```python
from build123d import *

# Parameters (mm, degrees)
ESBO_O1_W                   = 131.4
ESBO_O1_H                   = 68.4
BASE_DEPTH                  = 1.2
FILETE1_R                   = 15
FILETE2_R                   = 15
FILETE3_R                   = 10
FILETE4_R                   = 10
PAREDES_START               = 15.5
PAREDES_DEPTH               = 15.5
ESBO_O6_R                   = 2.5
SUPORTE_DOS_PARAFUSOS_DEPTH = 15.5
ESBO_O7_R                   = 1.1
FURO_DOS_PARAFUSOS_DEPTH    = 6
FECHAMENTOS_REACH           = 77.928
ESBO_O14_W                  = 10
ESBO_O14_H                  = 4.5
CORTE_DO_USB_DEPTH          = 10
ESBO_O16_W                  = 15.2
ESBO_O16_H                  = 9.3
CORTE_DAS_CHAVES_DEPTH      = 10
ESBO_O17_W                  = 15
ESBO_O17_H                  = 6
CORTE_SD_DEPTH              = 10
CHANFRO_BASE_INTERIOR_SIZE  = 2
FILETE5_R                   = 2


with BuildPart() as part:
    # Esboço1 → Base (new body)
    with BuildSketch(Plane(origin=(0, 0, 0), x_dir=(1, 0, 0), z_dir=(0, 1, 0))):
        Rectangle(ESBO_O1_W, ESBO_O1_H)
    extrude(amount=BASE_DEPTH)

    # Filete1
    filete1_edges = [part.edges().sort_by_distance(p)[0] for p in [
        (65.7, 0.6, 34.2),
    ]]
    fillet(filete1_edges, radius=FILETE1_R)

    # Filete2
    filete2_edges = [part.edges().sort_by_distance(p)[0] for p in [
        (-65.7, 0.6, 34.2),
    ]]
    fillet(filete2_edges, radius=FILETE2_R)

    # Filete3
    filete3_edges = [part.edges().sort_by_distance(p)[0] for p in [
        (65.7, 0.6, -34.2),
    ]]
    fillet(filete3_edges, radius=FILETE3_R)

    # Filete4
    filete4_edges = [part.edges().sort_by_distance(p)[0] for p in [
        (-65.7, 0.6, -34.2),
    ]]
    fillet(filete4_edges, radius=FILETE4_R)

    # Esboço5 → Paredes (add)
    with BuildSketch(Plane(origin=(0, 1.2, 0), x_dir=(1, 0, 0), z_dir=(0, 1, 0)).offset(PAREDES_START)):
        with BuildLine():
            Line((55.7, 34.2), (-55.7, 34.2))
            ThreePointArc((-55.7, 34.2), (-62.771067812, 31.271067812), (-65.7, 24.2))
            Line((-65.7, 24.2), (-65.7, -19.2))
            ThreePointArc((-65.7, -19.2), (-61.306601718, -29.806601718), (-50.7, -34.2))
            Line((-50.7, -34.2), (50.7, -34.2))
            ThreePointArc((50.7, -34.2), (61.306601718, -29.806601718), (65.7, -19.2))
            Line((65.7, -19.2), (65.7, 24.2))
            ThreePointArc((65.7, 24.2), (62.771067812, 31.271067812), (55.7, 34.2))
        make_face()
        with BuildLine():
            Line((55.7, 33), (-55.7, 33))
            ThreePointArc((-55.7, 33), (-61.922539674, 30.422539674), (-64.5, 24.2))
            Line((-64.5, 24.2), (-64.5, -19.2))
            ThreePointArc((-64.5, -19.2), (-60.45807358, -28.95807358), (-50.7, -33))
            Line((-50.7, -33), (50.7, -33))
            ThreePointArc((50.7, -33), (60.45807358, -28.95807358), (64.5, -19.2))
            Line((64.5, -19.2), (64.5, 24.2))
            ThreePointArc((64.5, 24.2), (61.922539674, 30.422539674), (55.7, 33))
        make_face(mode=Mode.SUBTRACT)
    extrude(amount=-PAREDES_DEPTH)

    # Esboço6 → Suporte dos parafusos (add)
    with BuildSketch(Plane(origin=(0, 1.2, 0), x_dir=(1, 0, 0), z_dir=(0, 1, 0))):
        with Locations(Location((-59.7, 28.2, 0), (0, 0, 90))):
            Circle(ESBO_O6_R)
        with Locations(Location((-57.7, -26.2, 0), (0, 0, 90))):
            Circle(ESBO_O6_R)
        with Locations(Location((59.7, 28.2, 0), (0, 0, 90))):
            Circle(ESBO_O6_R)
        with Locations(Location((57.7, -26.2, 0), (0, 0, 90))):
            Circle(ESBO_O6_R)
    extrude(amount=SUPORTE_DOS_PARAFUSOS_DEPTH)

    # Esboço7 → Furo dos parafusos (cut)
    with BuildSketch(Plane(origin=(0, 16.7, 0), x_dir=(1, 0, 0), z_dir=(0, 1, 0))):
        with Locations(Location((-59.7, 28.2, 0), (0, 0, 270))):
            Circle(ESBO_O7_R)
        with Locations(Location((59.7, 28.2, 0), (0, 0, 270))):
            Circle(ESBO_O7_R)
        with Locations(Location((57.7, -26.2, 0), (0, 0, 270))):
            Circle(ESBO_O7_R)
        with Locations(Location((-57.7, -26.2, 0), (0, 0, 270))):
            Circle(ESBO_O7_R)
    extrude(amount=-FURO_DOS_PARAFUSOS_DEPTH, mode=Mode.SUBTRACT)

    # Esboço23 → Fechamentos (add, up to next)
    with BuildSketch(Plane(origin=(0, 16.7, 0), x_dir=(1, 0, 0), z_dir=(0, 1, 0)), mode=Mode.PRIVATE) as fechamentos_sk1:
        with BuildLine():
            Line((57.2, 28.2), (57.2, 32.871216754))
            ThreePointArc((57.2, 32.871216754), (61.922539674, 30.422539674), (64.371216754, 25.7))
            Line((64.371216754, 25.7), (59.7, 25.7))
            Line((59.7, 25.7), (62.2, 28.2))
            Line((62.2, 28.2), (59.7, 30.7))
            Line((59.7, 30.7), (57.2, 28.2))
        make_face()
    fechamentos_tool1 = extrude(fechamentos_sk1.sketch, amount=-FECHAMENTOS_REACH, mode=Mode.PRIVATE) - part.part
    # Esboço23 → Fechamentos (add, up to next)
    with BuildSketch(Plane(origin=(0, 16.7, 0), x_dir=(1, 0, 0), z_dir=(0, 1, 0)), mode=Mode.PRIVATE) as fechamentos_sk2:
        with BuildLine():
            Line((-59.7, 25.7), (-64.371216754, 25.7))
            ThreePointArc((-64.371216754, 25.7), (-61.922539674, 30.422539674), (-57.2, 32.871216754))
            Line((-57.2, 32.871216754), (-57.2, 28.2))
            Line((-57.2, 28.2), (-59.7, 30.7))
            Line((-59.7, 30.7), (-62.2, 28.2))
            Line((-62.2, 28.2), (-59.7, 25.7))
        make_face()
    fechamentos_tool2 = extrude(fechamentos_sk2.sketch, amount=-FECHAMENTOS_REACH, mode=Mode.PRIVATE) - part.part
    # Esboço23 → Fechamentos (add, up to next)
    with BuildSketch(Plane(origin=(0, 16.7, 0), x_dir=(1, 0, 0), z_dir=(0, 1, 0)), mode=Mode.PRIVATE) as fechamentos_sk3:
        with BuildLine():
            Line((57.7, -23.7), (63.745688943, -23.7))
            ThreePointArc((63.745688943, -23.7), (60.45807358, -28.95807358), (55.2, -32.245688943))
            Line((55.2, -32.245688943), (55.2, -26.2))
            Line((55.2, -26.2), (57.7, -28.7))
            Line((57.7, -28.7), (60.2, -26.2))
            Line((60.2, -26.2), (57.7, -23.7))
        make_face()
    fechamentos_tool3 = extrude(fechamentos_sk3.sketch, amount=-FECHAMENTOS_REACH, mode=Mode.PRIVATE) - part.part
    # Esboço23 → Fechamentos (add, up to next)
    with BuildSketch(Plane(origin=(0, 16.7, 0), x_dir=(1, 0, 0), z_dir=(0, 1, 0)), mode=Mode.PRIVATE) as fechamentos_sk4:
        with BuildLine():
            Line((-55.2, -26.2), (-55.2, -32.245688943))
            ThreePointArc((-55.2, -32.245688943), (-60.45807358, -28.95807358), (-63.745688943, -23.7))
            Line((-63.745688943, -23.7), (-57.7, -23.7))
            Line((-57.7, -23.7), (-60.2, -26.2))
            Line((-60.2, -26.2), (-57.7, -28.7))
            Line((-57.7, -28.7), (-55.2, -26.2))
        make_face()
    fechamentos_tool4 = extrude(fechamentos_sk4.sketch, amount=-FECHAMENTOS_REACH, mode=Mode.PRIVATE) - part.part
    add(fechamentos_tool1.solids().sort_by_distance((57.301416, 16.7, -30.535608))[0])
    add(fechamentos_tool2.solids().sort_by_distance((-62.035608, 16.7, -25.801416))[0])
    add(fechamentos_tool3.solids().sort_by_distance((59.019684, 16.7, 27.519684))[0])
    add(fechamentos_tool4.solids().sort_by_distance((-59.019684, 16.7, 27.519684))[0])

    # Esboço14 → Corte do USB (cut)
    with BuildSketch(Plane(origin=(0, 0, -34.2), x_dir=(-1, 0, 0), z_dir=(0, 0, -1))):
        with Locations((48.7, 12.45)):
            Rectangle(ESBO_O14_W, ESBO_O14_H)
    extrude(amount=-CORTE_DO_USB_DEPTH, mode=Mode.SUBTRACT)

    # Esboço16 → Corte das chaves (cut)
    with BuildSketch(Plane(origin=(0, 0, -34.2), x_dir=(-1, 0, 0), z_dir=(0, 0, -1))):
        with Locations((-45.7, 8)):
            Rectangle(ESBO_O16_W, ESBO_O16_H)
        with Locations((-24.5, 8)):
            Rectangle(ESBO_O16_W, ESBO_O16_H)
    extrude(amount=-CORTE_DAS_CHAVES_DEPTH, mode=Mode.SUBTRACT)

    # Esboço17 → Corte SD (cut)
    with BuildSketch(Plane(origin=(65.7, 0, 0), x_dir=(0, 0, -1), z_dir=(1, 0, 0))):
        with Locations((6.2, 11)):
            Rectangle(ESBO_O17_W, ESBO_O17_H)
    extrude(amount=-CORTE_SD_DEPTH, mode=Mode.SUBTRACT)

    # Chanfro base interior
    chanfro_base_interior_edges = [part.edges().sort_by_distance(p)[0] for p in [
        (56.452759112, 1.2, -32.967745076),
        (-64.467745076, 1.2, -24.952759112),
        (64.310115859, 1.2, 21.481391306),
        (-52.981391306, 1.2, 32.810115859),
        (64.467745076, 1.2, -24.952759112),
        (0, 1.2, -33),
        (-56.452759112, 1.2, -32.967745076),
        (-64.5, 1.2, -2.5),
        (-64.310115859, 1.2, 21.481391306),
        (0, 1.2, 33),
        (52.981391306, 1.2, 32.810115859),
        (64.5, 1.2, -2.5),
    ]]
    chamfer(chanfro_base_interior_edges, length=CHANFRO_BASE_INTERIOR_SIZE)

    # Filete5
    # the kernel refuses this fillet: 2 mm, written as the material it adds along each edge
    with BuildSketch(Plane(origin=(64.371216754, 16.7, -25.7), x_dir=(0.06425854366242006, 0, 0.9979332841259403), z_dir=(0, -1, 0))) as filete5_piece_1_section:
        with BuildLine():
            CenterArc((1.875624905, 1.995866568), FILETE5_R, 183.684281821, 90)
            Line((-0.120241664, 1.867349481), (-0.31982832, 1.854497772))
            Line((-0.31982832, 1.854497772), (-0.199586657, -0.012851709))
            Line((-0.199586657, -0.012851709), (-0.021356822, -0.198856446))
            ThreePointArc((-0.021356822, -0.198856446), (1.518027059, -0.231715929), (2.016993701, -0.199586657))
            Line((2.016993701, -0.199586657), (2.004141992, 0))
        make_face()
    filete5_piece_1 = extrude(amount=18.51035498, mode=Mode.PRIVATE)
    filete5_piece_1 = split(filete5_piece_1, bisect_by=Plane(origin=(63.917041989, 0, -25.117041989), z_dir=(0, 1, 0)), keep=Keep.TOP, mode=Mode.PRIVATE)
    add(filete5_piece_1)


solid = part.part
```
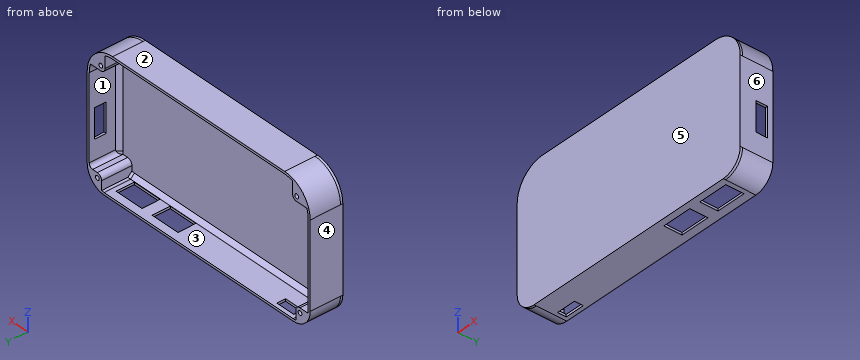
Model file for the job. Use its own axes, mm. Face numbers are marked on the shaded views. A direction names the side the tool comes from. Round coordinates to 2 decimals unless told otherwise and drop trailing zeros. Loops run counter-clockwise (first coordinate to the right, second up) from the corner with the lowest first, then second, coordinate; pieces in that order, holes last. Notation, with made-up numbers: M 77.25,57 L 117.25,57 A5 ccw 117.25,65 Z; hole C 1.5,-7.75 d7. An arc over 180 degrees is marked long. Put each result on its own line as item: value. Start each with the question number.
Item 1: Mould opens along X. For the marked faces 3, 4, 5 and 6 say: released by +X, released by -X, zero draft, split by the parting line, or undercut.
Item 2: Cut at B-B (x = -32.5). List the corners of the cut face in (y, z), then the cut area to 3 significant figures.
Item 3: Drill centre lines: line 1 along Z through (x, y) = (-30.5, 8.5); line 2 along X through (y, z) = (14.75, -14); line 3 along X through (y, z) = (12.8, -28.2). Where is each one in solid material? Low to high.
Item 4: Cut at C-C (z = 11). List the corners of the cut face in (x, y), then the cut area to 3 significant figures.
Item 5: Drop flat-ended pins along their axis: P1, Ø1, axis at x = 65, y = 10, coming from the -Z side; P2, Ø10, axis at x = 32, z = -18, coming from the +Y side; P3, Ø5, axis at y = 10.5, z = -30.5, coming from the -X side. Give the stop position or say it passes through.
Item 6: Cut at A-A (x = 48). List the corners of the cut face in (y, z).
Item 7: 3-axis set-ups, long thin cutter, end or side, ignore diameter. For the marked faces 1 and 2: which of +Z, -Z, +X, -X, +Y, -Y reach the whole face in a straight line?
Answer block:
1. face 3: undercut
1. face 4: released by -X
1. face 5: zero draft
1. face 6: released by +X
2. outline: M 0,-34.2 L 16.7,-34.2 L 16.7,-33 L 3.2,-33 L 1.2,-31 L 1.2,31 L 3.2,33 L 16.7,33 L 16.7,34.2 L 0,34.2 Z
2. area: 123 mm2
3. line 1: -34.2 to -33, 33 to 34.2
3. line 2: -65.7 to -64.5, 64.5 to 65.7
3. line 3: -64.87 to -60.8, -58.6 to -57.2, 57.2 to 58.6, 60.8 to 64.87
4. outline: M -65.7,0 L 65.7,0 L 65.7,16.7 L 64.5,16.7 L 64.5,3.2 L 62.5,1.2 L -62.5,1.2 L -64.5,3.2 L -64.5,16.7 L -65.7,16.7 Z
4. area: 199 mm2
5. P1: z = -28.95
5. P2: y = 1.2
5. P3: x = -64.95
6. outline: M 0,-34.2 L 3.35,-34.2 L 3.35,-33 L 3.2,-33 L 1.2,-31 L 1.2,31 L 3.2,33 L 16.7,33 L 16.7,34.2 L 0,34.2 Z; M 12.65,-34.2 L 16.7,-34.2 L 16.7,-33 L 12.65,-33 Z
7. face 1: +Y
7. face 2: +Z, +X, -X, +Y, -Y
